Read the model definition and answer for the solid it produces. Units are mm, in the model's axes. A direction names the side the tool comes from. Round coordinates to 2 decimals unless told otherwise and drop trailing zeros. Write each loop counter-clockwise with the first axis right and the second up, starting at its lowest first coordinate (ties: lowest second). Pieces come first, ordered by that corner, then holes. Notation, with made-up numbers: (-14.75, -37) -> (23.25, -37) arc R7 ccw to (23.25, -30) -> close; hole circle Ø3 at (12, 51.25). An arc over 180 degrees is marked (long way). Return JSON: item names as keys, results as strings. Group by question number.
(1) For faces 4 (the flat face through (-19, -39.594, 3)), 5 (the flat face through (-12.7, -20, 3)), 6 (the cylindrical face through (-0.689, 12.877, 3.131)), 7 (the flat face through (25.872, -23, 3)), 8 (the flat face through (-25.872, -24, 3)), determine the directions among +Z, -Z, +X, -X, +Y, -Y from which every point of the face is accessible in a straight line to the end or side of a thin tool.
(2) The mould has two halves that part along X. Classify faces 1 (the flat face through (1, 1, 0)), 2 (the flat face through (-38.015, 4.852, 3.131)), 3 (the flat face through (12.7, -20, 3)): released by +X, released by -X, zero draft, split by the parting line, or undercut.
(3) A cutting plane is placed at D-D on x = -37. Give the vertices of the cut face in (y, z), then the cut area to 3 significant figures.
(4) Straight lines are drawn through the part: line 1 (X direction, y = -32, z = 4.75); line 2 (Y direction, x = 19.05, z = 3.75); line 3 (X direction, y = -17.5, z = 1). For each, find the intervals that lie inside material, in ascending order.
(5) A cutting plane is placed at B-B on x = 19. Give the vertices of the cut face in (y, z).
(6) Given pin 1 (1.5 mm diameter, centred on y = -11, z = 5.5, fed in from -X); pin 2 (3 mm diameter, centred on y = -23.5, z = 2, fed in from +X); pin 3 (1.9 mm diameter, centred on x = 4, z = 3, fed in from -Y), each flat-ended and moving along its own axis, determine where each tip first touches the part or whether it passes through.
(7) A cutting plane is placed at A-A on y = -29.5. Give the vertices of the cut face in (x, z), then the cut area to 3 significant figures.
(8) A cutting plane is placed at C-C on z = 1.75. State how many separate pieces and enclosed holes the cut face has, then the cut area to 3 significant figures.
```python
from build123d import *

# Parameters (mm, degrees)
SKETCH1_R           = 1.905
SKETCH1_R_2         = 1.3890625
BOSS_EXTRUDE1_DEPTH = 6.35


with BuildPart() as part:
    # Sketch1 → Boss-Extrude1 (new body)
    with BuildSketch(Plane.XY):
        with BuildLine():
            Line((12.7, 0), (-12.7, 0))
            Line((-12.7, 0), (-12.7, -39.593860647))
            Line((-12.7, -39.593860647), (-25.872163348, -39.593860647))
            Line((-25.872163348, -39.593860647), (-25.872163348, -7.44555378))
            Line((-25.872163348, -7.44555378), (-50.502986928, 17.497884605))
            ThreePointArc((-50.502986928, 17.497884605), (-53.573053894, 23.997146119), (-46.71026588, 26.134399514))
            ThreePointArc((-46.71026588, 26.134399514), (0, 12.874711135), (46.71026588, 26.134399514))
            ThreePointArc((46.71026588, 26.134399514), (53.573053894, 23.997146119), (50.502986928, 17.497884605))
            Line((50.502986928, 17.497884605), (25.872163348, -7.44555378))
            Line((25.872163348, -7.44555378), (25.872163348, -39.593860647))
            Line((25.872163348, -39.593860647), (12.7, -39.593860647))
            Line((12.7, -39.593860647), (12.7, 0))
        make_face()
        with Locations((-19.05, -15.875)):
            Circle(SKETCH1_R, mode=Mode.SUBTRACT)
        with Locations(Location((19.05, -15.875, 0), (0, 0, 180))):
            Circle(SKETCH1_R, mode=Mode.SUBTRACT)
        with Locations((-49.2125, 22.082211135)):
            Circle(SKETCH1_R_2, mode=Mode.SUBTRACT)
        with Locations((-19.05, -34.925)):
            Circle(SKETCH1_R, mode=Mode.SUBTRACT)
        with Locations(Location((19.05, -34.925, 0), (0, 0, 180))):
            Circle(SKETCH1_R, mode=Mode.SUBTRACT)
        with Locations(Location((49.2125, 22.082211135, 0), (0, 0, 180))):
            Circle(SKETCH1_R_2, mode=Mode.SUBTRACT)
    extrude(amount=BOSS_EXTRUDE1_DEPTH)


solid = part.part
```
Checks:
{
 "1": {"face 4": "+Z, -Z, +X, -X, -Y", "face 5": "+Z, -Z, -Y", "face 6": "+Z, -Z, +Y", "face 7": "+Z, -Z, +X, -Y", "face 8": "+Z, -Z, -X, -Y"},
 "2": {"face 1": "zero draft", "face 2": "released by -X", "face 3": "undercut"},
 "3": {"outline": "(3.82, 0) -> (20.94, 0) -> (20.94, 6.35) -> (3.82, 6.35) -> close", "area": "109 mm^2"},
 "4": {"line 1": "x = -25.87 to -12.7, 12.7 to 25.87", "line 2": "y = -39.59 to -36.83, -33.02 to -17.78, -13.97 to 14.94", "line 3": "x = -25.87 to -20.04, -18.06 to -12.7, 12.7 to 18.06, 20.04 to 25.87"},
 "5": {"outline": "(-39.59, 0) -> (-36.83, 0) -> (-36.83, 6.35) -> (-39.59, 6.35) -> close; (-33.02, 0) -> (-17.78, 0) -> (-17.78, 6.35) -> (-33.02, 6.35) -> close; (-13.97, 0) -> (14.93, 0) -> (14.93, 6.35) -> (-13.97, 6.35) -> close"},
 "6": {"pin 1": "stops at x = -25.87", "pin 2": "stops at x = 25.87", "pin 3": "stops at y = 0"},
 "7": {"outline": "(-25.87, 0) -> (-12.7, 0) -> (-12.7, 6.35) -> (-25.87, 6.35) -> close; (12.7, 0) -> (25.87, 0) -> (25.87, 6.35) -> (12.7, 6.35) -> close", "area": "167 mm^2"},
 "8": {"separate pieces": "1", "enclosed holes": "6", "area": "2,590 mm^2"}
}
